from build123d import *


with BuildPart() as part:
    # Sketch2 → Revolve1 (revolve)
    with BuildSketch(Plane(origin=(0, 0, 0), x_dir=(0, 1, 0), z_dir=(0, 0, 1)), mode=Mode.PRIVATE) as revolve1_sk:
        Polygon((0, 43.554), (0, 29.1925), (0, 27.2875), (20, 27.2875), (20, 43.554), align=None)
        Polygon((0, 49.972526435), (-9.525, 49.972526435), (-9.525, 29.1925), (0, 29.1925), (0, 43.554), align=None)
        Polygon((20, 27.2875), (50, 43.554), (20, 43.554), align=None)
    revolve(revolve1_sk.sketch.rotate(Axis((0, 52.97625, 0), (0, -1, 0)), 270), axis=Axis((0, 52.97625, 0), (0, -1, 0)))


solid = part.part
Geometry check sheet. Reference: the model listing, model coordinates, mm. A direction names the side the tool comes from. Give positions to 0.01 mm unless a question says otherwise; leave off trailing zeros. Order: outer loops, then holes, each group sorted by start corner. A loop starts at its lowest first (then second) coordinate and runs counter-clockwise, first axis right, second up.
1) Tool access check on faces 4 (the cylindrical face through (-8.769, -4.696, 27.844)), 5 (the flat face through (-45, 0, -3)), 6 (the cylindrical face through (-27.055, 10.14, -3.552)). Record the directions out of +Z, -Z, +X, -X, +Y, -Y that give a thin tool (end or side, any length) a straight path to the whole face; none if there is none.
Results are:
face 4: -Y
face 5: +Y
face 6: +Y, -Y
2) Cross-section at A-A (z = 0). Record the boundary of the cut face in (x, y) (1 decimal), then the cut area to 3 significant figures.
Results are:
outline: (-50, -9.5) - (-29.2, -9.5) - (-29.2, 0) - (-27.3, 0) - (-27.3, 20) - (-43.6, 50) - (-43.6, 0) - (-50, 0) - close; (27.3, 0) - (29.2, 0) - (29.2, -9.5) - (50, -9.5) - (50, 0) - (43.6, 0) - (43.6, 50) - (27.3, 20) - close
area: 1,530 mm2
3) Material ranges on probe 1 along X at (y, z) = (-4, 0); probe 2 along X at (y, z) = (8.75, 0); probe 3 along Z at (x, y) = (-20, 28), recorded low to high.
Results are:
probe 1: x = -49.97 to -29.19, 29.19 to 49.97
probe 2: x = -43.55 to -27.29, 27.29 to 43.55
probe 3: z = -38.69 to -24.5, 24.5 to 38.69
4) Cross-section at D-D (y = 29.5). Record the boundary of the cut face in (x, z), then the cut area to 3 significant figures.
Results are:
outline: circle Ø87.11 at (0, 0); hole circle Ø64.88 at (0, 0)
area: 2,650 mm2
5) Draft check along X on faces 1 (the flat face through (21.5, 0, 17.2)), 2 (the cylindrical face through (44.334, -4.829, 23.059)), 3 (the flat face through (22, -9.525, 22)). Enter one of: released by +X, released by -X, zero draft, split by the parting line, or undercut.
Results are:
face 1: undercut
face 2: split by the parting line
face 3: zero draft
6) Cross-section at C-C (y = 9). Record the boundary of the cut face in (x, z) (1 decimal).
Results are:
outline: circle Ø87.1 at (0, 0); hole circle Ø54.6 at (0, 0)
7) Cross-section at B-B (x = 0). Record the boundary of the cut face in (y, z) (1 decimal).
Results are:
outline: (-9.5, -50) - (0, -50) - (0, -43.6) - (50, -43.6) - (20, -27.3) - (0, -27.3) - (0, -29.2) - (-9.5, -29.2) - close; (-9.5, 29.2) - (0, 29.2) - (0, 27.3) - (20, 27.3) - (50, 43.6) - (0, 43.6) - (0, 50) - (-9.5, 50) - close
8) Gauge pin test, flat ends, axial feed: pin 1 (6 mm diameter, centred on x = -0.5, y = 7.5, fed in from +Z); pin 2 (2 mm diameter, centred on y = 42, z = -7, fed in from -X); pin 3 (3 mm diameter, centred on x = 27.5, z = 0, fed in from +Y). Record the tip position at first contact, or that the pin passes through.
Results are:
pin 1: stops at z = 43.55
pin 2: stops at x = -43.14
pin 3: stops at y = 23.16
